Could you check a few things on this model? Use its own coordinates, in mm. A direction names the side the tool comes from. Coordinates: 2 decimals unless noted, no trailing zeros. Order: outer loops, then holes, each group sorted by start corner. A loop starts at its lowest first (then second) coordinate and runs counter-clockwise, first axis right, second up. Notation, with made-up numbers: (78, 24.25) -> (88, 24.25) arc R10 cw to (88, 38.25) -> close; hole circle Ø8 at (54, 83). An arc over 180 degrees is marked (long way). Return JSON: item names as keys, results as strings. Group by question number.
from build123d import *

# Parameters (mm, degrees)
F0_W     = 38.1
F0_H     = 19.05
F1_DEPTH = 698.5
F3_DEPTH = 698.501


with BuildPart() as f1:
    # F0 (on Front) → F1 (new body)
    with BuildSketch(Plane.XZ):
        Rectangle(F0_W, F0_H)
    extrude(amount=F1_DEPTH)

    # F2 (on face) → F3 (cut, through all)
    with BuildSketch(Plane.XZ.offset(698.5)):
        Polygon((-19.05, 0), (-19.05, -3.175), (-7.569117, -3.175), (-7.569117, 3.175), (-19.05, 3.175), align=None)
    extrude(amount=-F3_DEPTH, mode=Mode.SUBTRACT)


solid = f1.part
Q1. I want a section at A-A on y = -361.5. Please give me the cut outline in (x, z) (3 decimals).
Q2. We'd pull the mould along Z, two halves only. Please class faces 3 (the flat face through (0, -344, -9.525)), 4 (the flat face through (0, 0, 0)), 5 (the flat face through (-13, -354, -3.175)): pulls with the +Z half, pulls with the -Z half, needs draft (parallel to the pull), parting line crosses it, or undercut.
Q3. I need wall thicknesses on line 1 along Z through (x, y) = (-14.5, -241.5) (3 decimals); line 2 along X through (y, z) = (-216.5, -1.75). Which ranges of each line are inside material? Lowest first, please. Write a range as from..to.
Q4. I'm going to push a flat-ended pin straight in: pin 1 Ø3 at (y, z) = (-207.5, 1.5) entering from -X. Where does the tip first touch, or does it pass through?
Q5. On a 3-axis mill with a long thin cutter (end or side, diameter ignored), from which of +Z, -Z, +X, -X, +Y, -Y can I reach the whole of each face in a straight line? I mean faces 1 (the flat face through (0, -344, 9.525)), 2 (the flat face through (-13, -354, 3.175)). Say none if no direction works.
Response values:
{
 "1": {"outline": "(-19.05, -9.525) -> (19.05, -9.525) -> (19.05, 9.525) -> (-19.05, 9.525) -> (-19.05, 3.175) -> (-7.569, 3.175) -> (-7.569, -3.175) -> (-19.05, -3.175) -> close"},
 "2": {"face 3": "pulls with the -Z half", "face 4": "needs draft", "face 5": "undercut"},
 "3": {"line 1": "z = -9.525..-3.175, 3.175..9.525", "line 2": "x = -7.57..19.05"},
 "4": {"pin 1": "stops at x = -7.57"},
 "5": {"face 1": "+Z, +X, -X, +Y, -Y", "face 2": "-X, +Y, -Y"}
}
